Could you check a few things on this model? Use its own coordinates, in mm. Face numbers are marked on the shaded views. A direction names the side the tool comes from. Coordinates: 2 decimals unless noted, no trailing zeros. Order: outer loops, then holes, each group sorted by start corner. A loop starts at its lowest first (then second) coordinate and runs counter-clockwise, first axis right, second up. Notation, with made-up numbers: (-29.75, 35.5) - (29.25, 35.5) arc R28 ccw to (29.25, 57.5) - close; hole circle Ø6 at (-1.75, 62). An arc over 180 degrees is marked (long way). One line per item, written item: value.
Autodesk Inventor part; units mm, degrees
ref_plane "YZ Plane" through (0, 0, 0) normal (1, 0, 0) x (0, 1, 0)
ref_plane "XZ Plane" through (0, 0, 0) normal (0, 1, 0) x (-1, 0, 0)
ref_plane "XY Plane" through (0, 0, 0) normal (0, 0, 1) x (1, 0, 0)
sketch "Sketch_1" plane through (0, 0, 0) normal (0, 0, 1) x (1, 0, 0)
  arc A0 (-8, -1.5757) -> (-7.9121, -1.7879) centre (-7.7, -1.5757) ccw
  line L0 (-7.9121, -1.7879) -> (-5.5879, -4.1121)
  arc A1 (-5.5879, -4.1121) -> (-5.3757, -4.2) centre (-5.3757, -3.9) ccw
  line L1 (-5.3757, -4.2) -> (5.3757, -4.2)
  arc A2 (5.3757, -4.2) -> (5.5879, -4.1121) centre (5.3757, -3.9) ccw
  line L2 (5.5879, -4.1121) -> (7.9121, -1.7879)
  arc A3 (7.9121, -1.7879) -> (8, -1.5757) centre (7.7, -1.5757) ccw
  line L3 (8, -1.5757) -> (8, -0.3)
  arc A4 (8, -0.3) -> (7.7, 0) centre (7.7, -0.3) ccw
  line L4 (7.7, 0) -> (4.2, 0)
  arc A5 (3.9, 0.3) -> (4.2, 0) centre (4.2, 0.3) ccw
  line L5 (3.9, 0.3) -> (3.9, 1.5)
  arc A6 (3.9, 1.5) -> (3.6, 1.8) centre (3.6, 1.5) ccw
  line L6 (3.6, 1.8) -> (0.75, 1.8)
  line L7 (0.75, 1.8) -> (0.1124, 1.5424)
  arc A7 (-0.1124, 1.5424) -> (0.1124, 1.5424) centre (0, 1.8205) ccw
  line L8 (-0.1124, 1.5424) -> (-0.75, 1.8)
  line L9 (-0.75, 1.8) -> (-3.6, 1.8)
  arc A8 (-3.6, 1.8) -> (-3.9, 1.5) centre (-3.6, 1.5) ccw
  line L10 (-3.9, 1.5) -> (-3.9, 0.3)
  arc A9 (-4.2, 0) -> (-3.9, 0.3) centre (-4.2, 0.3) ccw
  line L11 (-4.2, 0) -> (-7.7, 0)
  arc A10 (-7.7, 0) -> (-8, -0.3) centre (-7.7, -0.3) ccw
  line L12 (-8, -0.3) -> (-8, -1.5757)
extrude "Extrusion1" add sketch "Sketch_1" along normal mid plane 16
sketch "Sketch_2" plane through (0, 0, 0) normal (1, 0, 0) x (0, 1, 0)
  line L0 (1.8, 0) -> (-4.2, 0)
  line L1 (-4.2, 0) -> (-4.2, 2)
  line L2 (-4.2, 2) -> (-3.821, 1.621)
  line L3 (-3.821, 1.621) -> (1.421, 1.621)
  line L4 (1.421, 1.621) -> (1.8, 2)
  line L5 (1.8, 2) -> (1.8, 0)
  line L6 (1.8, 0) -> (-4.2, 0)
revolve "Revolution1" cut sketch "Sketch_2" angle 360 about axis through (0, 1.8, 0) along (0, 1, 0)
thread "Thread1"
properties part number "13022_m"
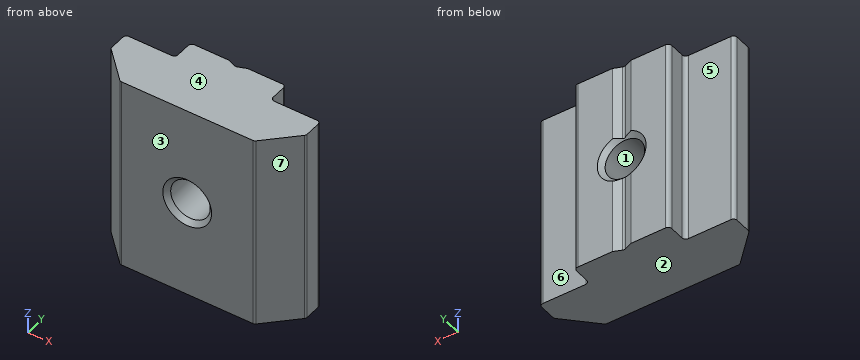
Item 1: If I drill on probe 1 along X at (y, z) = (-0.55, 0); probe 2 along Y at (x, z) = (4.75, 0.25); probe 3 along X at (y, z) = (0.75, -5), over which ranges is the centre line in solid material (lowest first)?
Conclusion:
probe 1: -8 to -1.62, 1.62 to 8
probe 2: -4.2 to 0
probe 3: -3.9 to 3.9
Item 2: Thinking about a two-plate mould opening in Z: for the marked faces 1, 2, 3 and 4, which applies, pulls with the +Z half, pulls with the -Z half, needs draft (parallel to the pull), parting line crosses it, or undercut?
Conclusion:
face 1: undercut
face 2: pulls with the -Z half
face 3: needs draft
face 4: pulls with the +Z half
Item 3: I want a section at A-A on z = 0. Please give me the cut outline in (x, y), then the cut area to 3 significant figures.
Conclusion:
outline: (-8, -1.58) arc R0.3 ccw to (-7.91, -1.79) - (-5.59, -4.11) arc R0.3 ccw to (-5.38, -4.2) - (-2, -4.2) - (-1.62, -3.82) - (-1.62, 1.42) - (-2, 1.8) - (-3.6, 1.8) arc R0.3 ccw to (-3.9, 1.5) - (-3.9, 0.3) arc R0.3 cw to (-4.2, 0) - (-7.7, 0) arc R0.3 ccw to (-8, -0.3) - close; (1.62, -3.82) - (2, -4.2) - (5.38, -4.2) arc R0.3 ccw to (5.59, -4.11) - (7.91, -1.79) arc R0.3 ccw to (8, -1.58) - (8, -0.3) arc R0.3 ccw to (7.7, 0) - (4.2, 0) arc R0.3 cw to (3.9, 0.3) - (3.9, 1.5) arc R0.3 ccw to (3.6, 1.8) - (2, 1.8) - (1.62, 1.42) - close
area: 55.2 mm²
Item 4: I want a section at C-C on y = -3. Please give me the cut outline in (x, z), then the cut area to 3 significant figures.
Conclusion:
outline: (-6.7, -8) - (6.7, -8) - (6.7, 8) - (-6.7, 8) - close; hole circle Ø3.24 at (0, 0)
area: 206 mm²
Item 5: For the marked faces 5, 6 and 7, which set-ups out of +Z, -Z, +X, -X, +Y, -Y let a thin tool reach every point of the face, with its end or its side?
Conclusion:
face 5: +Z, -Z, -X, +Y
face 6: +Z, -Z, +X, +Y
face 7: +Z, -Z, +X, -Y
Item 6: I'm going to push flat-ended pins straight in: pin 1 Ø1.5 at (y, z) = (0.5, 4.5) entering from -X; pin 2 Ø4 at (x, z) = (-6.5, -1) entering from +Y. Where does each tip first touch, or does it pass through?
Conclusion:
pin 1: x = -8
pin 2: y = 0
Item 7: I want a section at B-B on z = 5. Please give me the cut outline in (x, y).
Conclusion:
outline: (-8, -1.58) arc R0.3 ccw to (-7.91, -1.79) - (-5.59, -4.11) arc R0.3 ccw to (-5.38, -4.2) - (5.38, -4.2) arc R0.3 ccw to (5.59, -4.11) - (7.91, -1.79) arc R0.3 ccw to (8, -1.58) - (8, -0.3) arc R0.3 ccw to (7.7, 0) - (4.2, 0) arc R0.3 cw to (3.9, 0.3) - (3.9, 1.5) arc R0.3 ccw to (3.6, 1.8) - (0.75, 1.8) - (0.11, 1.54) arc R0.3 cw to (-0.11, 1.54) - (-0.75, 1.8) - (-3.6, 1.8) arc R0.3 ccw to (-3.9, 1.5) - (-3.9, 0.3) arc R0.3 cw to (-4.2, 0) - (-7.7, 0) arc R0.3 ccw to (-8, -0.3) - close
Item 8: I want a section at D-D on y = -2. Please give me the cut outline in (x, z).
Conclusion:
outline: (-7.7, -8) - (7.7, -8) - (7.7, 8) - (-7.7, 8) - close; hole circle Ø3.24 at (0, 0)
